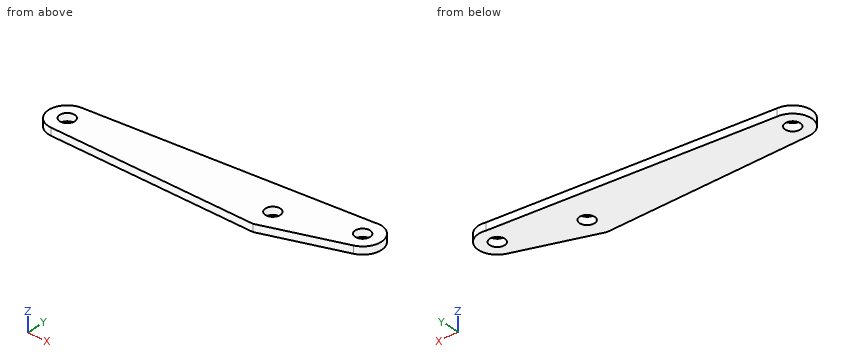
from build123d import *

# Parameters (mm, degrees)
CROQUIS1_R              = 4
SALIENTE_EXTRUIR1_DEPTH = 4


with BuildPart() as part:
    # Croquis1 → Saliente-Extruir1 (new body)
    # profile 1 of 2: a face of its own
    with BuildSketch(Plane.XY):
        with BuildLine():
            Line((0, -12.5), (42.408285537, 1.768055956))
            ThreePointArc((42.408285537, 1.768055956), (48.843358342, 13.962787444), (36.981350661, 20.992325968))
            Line((36.981350661, 20.992325968), (0, 12.5))
            Line((0, 12.5), (-112.222936903, 9.997514648))
            ThreePointArc((-112.222936903, 9.997514648), (-122, 0), (-112.222936903, -9.997514648))
            Line((-112.222936903, -9.997514648), (0, -12.5))
        make_face()
        with Locations((-112, 0)):
            Circle(CROQUIS1_R, mode=Mode.SUBTRACT)
        with Locations((39.219477194, 11.246004117)):
            Circle(CROQUIS1_R, mode=Mode.SUBTRACT)
        Circle(CROQUIS1_R, mode=Mode.SUBTRACT)
    # profile 2 of 2: a face of its own
    with BuildSketch(Plane.XY):
        Polygon((-112.222936903, 9.997514648), (36.981350661, 20.992325968), (0, 12.5), align=None)
    extrude(amount=SALIENTE_EXTRUIR1_DEPTH)


solid = part.part
Can you work these out from the model? Positions are in its coordinate system, mm. Coordinates: 2 decimals unless noted, no trailing zeros. Order: outer loops, then holes, each group sorted by start corner. A loop starts at its lowest first (then second) coordinate and runs counter-clockwise, first axis right, second up. Notation, with made-up numbers: M 21.25,13.5 L 35.25,13.5 A16 ccw 35.25,31.5 Z; hole C -11,54 d11. An arc over 180 degrees is marked long. Write item = value, one per line.
(1) Suppose I cut it at C-C on x = -96. Please give me the cut outline in (y, z).
Results are:
outline = M -10.36,0 L 11.19,0 L 11.19,4 L -10.36,4 Z
(2) Suppose I cut it at A-A on z = 2.45. Please give me the cut outline in (x, y).
Results are:
outline = M -112.22,-10 L 0,-12.5 L 42.41,1.77 A10 ccw 36.98,20.99 L -112.22,10 A10 ccw Z; hole C -112,0 d8; hole C 0,0 d8; hole C 39.22,11.25 d8
(3) For pin 1 Ø7 at (x, y) = (-112, 0) entering from -Z; pin 2 Ø1 at (x, z) = (-44.5, 1.5) entering from +Y; pin 3 Ø1.5 at (x, z) = (-12, 2.5) entering from -Y, each with a flat end and sliding along its axis, tell me the tip position at first contact or that it passes through.
Results are:
pin_1 = through
pin_2 = 15.02
pin_3 = -12.25
(4) Suppose I cut it at B-B on y = 0. Please give me the cut outline in (x, z).
Results are:
outline = M -122,0 L -116,0 L -116,4 L -122,4 Z; M -108,0 L -4,0 L -4,4 L -108,4 Z; M 4,0 L 37.15,0 L 37.15,4 L 4,4 Z
(5) Suppose I cut it at D-D on x = -25. Please give me the cut outline in (y, z), plus the area to 3 significant figures.
Results are:
outline = M -11.94,0 L 16.42,0 L 16.42,4 L -11.94,4 Z
area = 113 mm2
(6) I need wall thicknesses on line 1 along Y through (x, z) = (-112, 1.5); line 2 along X through (y, z) = (3, 1.05); line 3 along Y through (x, z) = (0, 1.4). Which ranges of each line are inside material? Lowest first, please. Write a range as [from, to].
Results are:
line_1 = [-10, -4], [4, 10.01]
line_2 = [-121.54, -114.65], [-109.35, -2.65], [2.65, 44.88]
line_3 = [-12.5, -4], [4, 18.27]
